Here's how the part is built. I have some questions about the finished solid (model axes, mm). A direction names the side the tool comes from. Coordinates: 2 decimals unless noted, no trailing zeros. Order: outer loops, then holes, each group sorted by start corner. A loop starts at its lowest first (then second) coordinate and runs counter-clockwise, first axis right, second up. Notation, with made-up numbers: (-28.75, 79.25) - (9.25, 79.25) arc R21 ccw to (9.25, 84.25) - close; hole circle Ø4 at (63, 49). An arc over 180 degrees is marked (long way). Answer as CSV lines item,"result". Start each with the question number.
Item 1: On a 3-axis mill with a long thin cutter (end or side, diameter ignored), from which of +Z, -Z, +X, -X, +Y, -Y can I reach the whole of each face in a straight line? I mean faces 1 (the face through (126, 2.478, 125)), 2 (the face through (0, -25, -20.408)), 3 (the face through (0, -12.729, 0)). Say none if no direction works.
Item 2: I need wall thicknesses on line 1 (X direction, y = 2, z = 37); line 2 (Y direction, x = 130, z = 122); line 3 (Y direction, x = 79, z = 74). Which ranges of each line are inside material? Lowest first, please.
Item 3: Imagine slicing it at B-B on z = 67. List the corners of the cut face in (x, y) for me.
Item 4: We'd pull the mould along X, two halves only. Please class faces 4 (the face through (22.5, -13, 2)), 5 (the face through (138.36, 4.94, -139.18)), 6 (the face through (0, -27.522, 0)), 7 (the face through (87.27, 1.21, -83.48)): pulls with the +X half, pulls with the -X half, needs draft (parallel to the pull), parting line crosses it, or undercut.
Item 5: I'm going to push flat-ended pins straight in: pin 1 (22 mm diameter, centred on y = -7, z = -6, fed in from -X); pin 2 (12 mm diameter, centred on y = -9.5, z = 32.5, fed in from -X); pin 3 (5 mm diameter, centred on y = -22.5, z = 5.5, fed in from +X); pin 4 (6 mm diameter, centred on x = 0, y = -21.5, fed in from -Z). Where does each tip first touch, or does it pass through?
Item 6: Imagine slicing it at A-A on z = 6. Count the separate pieces of the cut face and the enclosed holes in it, and give its area (3 significant figures).
from build123d import *

# Parameters (mm, degrees)
EXTRUDE_1_DEPTH     = 5
SKETCH_2_W          = 90
SKETCH_2_H          = 90
EXTRUDE_2_DEPTH     = 25
SKETCH_3_W          = 82.667839838
SKETCH_3_H          = 15.058257345
CUT_EXTRUDE_1_DEPTH = 90
SKETCH_4_W          = 82.085695662
SKETCH_4_H          = 16.995101666
CUT_EXTRUDE_2_DEPTH = 90
SKETCH_5_W          = 97.364780094
SKETCH_5_H          = 98.94366842
EXTRUDE_3_DEPTH     = 20
FILLET_1_R          = 10
SKETCH_6_W          = 90
SKETCH_6_H          = 90
EXTRUDE_4_DEPTH     = 30
CUT_EXTRUDE_3_DEPTH = 90
SKETCH_8_W          = 62.667839838
SKETCH_8_H          = 13.124346315
CUT_EXTRUDE_4_DEPTH = 10
CUT_EXTRUDE_5_DEPTH = 90
SKETCH_10_W         = 62.085695662
SKETCH_10_H         = 21.626220655
CUT_EXTRUDE_6_DEPTH = 10
SKETCH_11_W         = 62.667839838
SKETCH_11_H         = 13.124346315
CUT_EXTRUDE_7_DEPTH = 10
SKETCH_12_W         = 62.085695662
SKETCH_12_H         = 21.626220655
CUT_EXTRUDE_8_DEPTH = 10
EXTRUDE_5_DEPTH     = 20
SKETCH_14_R         = 25
EXTRUDE_6_DEPTH     = 20
FILLET_2_R          = 10
SCALE_1_SCALE       = 0.5


with BuildPart() as part:
    # 草图1 → 凸台-拉伸1 (new body)
    with BuildSketch(Plane(origin=(0, 0, 0), x_dir=(1, 0, 0), z_dir=(0, 1, 0))):
        Polygon((0, 70.903454713), (0, 0), (70.90345471, 0), (70.90345471, 50.896669322), (70.90345471, 63.546624398), (70.90345471, 70.903454713), (63.546624395, 70.903454713), (50.896669319, 70.903454713), align=None)
        Polygon((72.962659229, 92.969444623), (50.896669319, 70.903454713), (63.546624395, 70.903454713), (79.287636767, 86.644467085), align=None)
        Polygon((70.90345471, 70.903454713), (70.90345471, 63.546624398), (86.644467082, 79.28763677), (79.287636767, 86.644467085), (63.546624395, 70.903454713), align=None)
        Polygon((70.90345471, 63.546624398), (70.90345471, 50.896669322), (92.96944462, 72.962659232), (86.644467082, 79.28763677), align=None)
        with BuildLine():
            ThreePointArc((242.661241038, 250.018071355), (240.67172678, 254.833829646), (239.993214606, 260))
            Line((239.993214606, 260), (72.962659229, 92.969444623))
            Line((72.962659229, 92.969444623), (79.287636767, 86.644467085))
            Line((79.287636767, 86.644467085), (242.661241038, 250.018071355))
        make_face()
        with BuildLine():
            Line((92.96944462, 72.962659232), (260, 239.993214612))
            ThreePointArc((260, 239.993214606), (254.833829644, 240.67172678), (250.018071352, 242.66124104))
            Line((250.018071352, 242.66124104), (86.644467082, 79.28763677))
            Line((86.644467082, 79.28763677), (92.96944462, 72.962659232))
        make_face()
        with BuildLine():
            Line((260, 252.643169688), (260, 239.993214612))
            ThreePointArc((260, 239.993214606), (274.146933622, 245.853066378), (280.006785394, 260))
            ThreePointArc((280.006785394, 260), (260, 280.006785394), (239.993214606, 260))
            Line((239.993214606, 260), (252.643169682, 260))
            Line((252.643169682, 260), (260, 260))
            Line((260, 260), (260, 252.643169688))
        make_face()
        with BuildLine():
            Line((252.643169682, 260), (239.993214606, 260))
            ThreePointArc((239.993214606, 260), (240.67172678, 254.833829646), (242.661241038, 250.018071355))
            Line((242.661241038, 250.018071355), (252.643169682, 260))
        make_face()
        with BuildLine():
            ThreePointArc((250.018071352, 242.66124104), (254.833829644, 240.67172678), (260, 239.993214606))
            Line((260, 239.993214612), (260, 252.643169688))
            Line((260, 252.643169688), (250.018071352, 242.66124104))
        make_face()
    extrude_1 = extrude(amount=EXTRUDE_1_DEPTH)

    # 镜向1: 凸台-拉伸1 across plane
    add(extrude_1.mirror(Plane(origin=(0, 5, 0), x_dir=(0, 0, 1), z_dir=(1, 0, 0))))

    # 镜向3: part across plane


with BuildPart() as part_1:
    add(part.part)
    add(part.part.mirror(Plane(origin=(0, 5, 0), x_dir=(1, 0, 0), z_dir=(0, 0, -1))))

    # 草图2 → 凸台-拉伸2 (add)
    with BuildSketch(Plane.XZ):
        Rectangle(SKETCH_2_W, SKETCH_2_H)
    extrude(amount=EXTRUDE_2_DEPTH)

    # 草图3 → 切除-拉伸1 (cut)
    with BuildSketch(Plane.XY.offset(45)):
        with Locations((0, -12.246888496)):
            Rectangle(SKETCH_3_W, SKETCH_3_H)
    extrude(amount=-CUT_EXTRUDE_1_DEPTH, mode=Mode.SUBTRACT)

    # 草图4 → 切除-拉伸2 (cut)
    with BuildSketch(Plane(origin=(45, 0, 0), x_dir=(0, 0, -1), z_dir=(1, 0, 0))):
        with Locations((0, -12.272398252)):
            Rectangle(SKETCH_4_W, SKETCH_4_H)
    extrude(amount=-CUT_EXTRUDE_2_DEPTH, mode=Mode.SUBTRACT)

    # 草图5 → 凸台-拉伸3 (add)
    with BuildSketch(Plane(origin=(0, 5, 0), x_dir=(1, 0, 0), z_dir=(0, 1, 0))):
        Rectangle(SKETCH_5_W, SKETCH_5_H)
    extrude(amount=EXTRUDE_3_DEPTH)

    # 圆角1
    fillet_1_edges = [part_1.edges().sort_by_distance(p)[0] for p in [
        (48.682390047, 15, 49.47183421),
        (48.682390047, 15, -49.47183421),
        (-48.682390047, 15, -49.47183421),
        (-48.682390047, 15, 49.47183421),
        (48.682390047, 25, 0),
        (0, 25, -49.47183421),
        (-48.682390047, 25, 0),
        (0, 25, 49.47183421),
    ]]
    fillet(fillet_1_edges, radius=FILLET_1_R)

    # 草图6 → 凸台-拉伸4 (add)
    with BuildSketch(Plane.XZ.offset(25)):
        Rectangle(SKETCH_6_W, SKETCH_6_H)
    extrude(amount=EXTRUDE_4_DEPTH)

    # 草图7 → 切除-拉伸3 (cut)
    with BuildSketch(Plane.XY.offset(45)):
        Polygon((-41.333919919, -25.414932676), (41.333919919, -25.414932676), (41.333919919, -49.347564191), (31.333919919, -49.347564191), (31.333919919, -36.223217876), (-31.333919919, -36.223217876), (-31.333919919, -49.347564191), (-41.333919919, -49.347564191), align=None)
    extrude(amount=-CUT_EXTRUDE_3_DEPTH, mode=Mode.SUBTRACT)

    # 草图8 → 切除-拉伸4 (cut)
    with BuildSketch(Plane.XY.offset(45)):
        with Locations((0, -42.785391034)):
            Rectangle(SKETCH_8_W, SKETCH_8_H)
    extrude(amount=-CUT_EXTRUDE_4_DEPTH, mode=Mode.SUBTRACT)

    # 草图9 → 切除-拉伸5 (cut)
    with BuildSketch(Plane(origin=(45, 0, 0), x_dir=(0, 0, -1), z_dir=(1, 0, 0))):
        Polygon((-41.042847831, -26.273596919), (-41.042847831, -50.943507888), (-31.042847831, -50.943507888), (-31.042847831, -29.317287233), (31.042847831, -29.317287233), (31.042847831, -50.943507888), (41.042847831, -50.943507888), (41.042847831, -26.273596919), align=None)
    extrude(amount=-CUT_EXTRUDE_5_DEPTH, mode=Mode.SUBTRACT)

    # 草图10 → 切除-拉伸6 (cut)
    with BuildSketch(Plane(origin=(45, 0, 0), x_dir=(0, 0, -1), z_dir=(1, 0, 0))):
        with Locations((0, -40.130397561)):
            Rectangle(SKETCH_10_W, SKETCH_10_H)
    extrude(amount=-CUT_EXTRUDE_6_DEPTH, mode=Mode.SUBTRACT)

    # 草图11 → 切除-拉伸7 (cut)
    with BuildSketch(Plane(origin=(0, 0, -45), x_dir=(-1, 0, 0), z_dir=(0, 0, -1))):
        with Locations((0, -42.785391034)):
            Rectangle(SKETCH_11_W, SKETCH_11_H)
    extrude(amount=-CUT_EXTRUDE_7_DEPTH, mode=Mode.SUBTRACT)

    # 草图12 → 切除-拉伸8 (cut)
    with BuildSketch(Plane.ZY.offset(45)):
        with Locations((0, -40.130397561)):
            Rectangle(SKETCH_12_W, SKETCH_12_H)
    extrude(amount=-CUT_EXTRUDE_8_DEPTH, mode=Mode.SUBTRACT)

    # 草图13 → 凸台-拉伸5 (add)
    with BuildSketch(Plane.XY.offset(70.903454713)):
        Polygon((0, 0), (-10, 0), (-10, 5), (10, 5), (10, 0), align=None)
    extrude(amount=EXTRUDE_5_DEPTH)

    # 草图14 → 凸台-拉伸6 (add)
    with BuildSketch(Plane(origin=(0, 5, 0), x_dir=(1, 0, 0), z_dir=(0, 1, 0))):
        with Locations(Location((-260, 260, 0), (0, 0, 349.463237906))):
            Circle(SKETCH_14_R)
        with Locations(Location((260, 260, 0), (0, 0, 190.536762094))):
            Circle(SKETCH_14_R)
        with Locations(Location((-260, -260, 0), (0, 0, 79.463237895))):
            Circle(SKETCH_14_R)
        with Locations(Location((260, -260, 0), (0, 0, 100.536762105))):
            Circle(SKETCH_14_R)
    extrude(amount=EXTRUDE_6_DEPTH)

    # 圆角2
    fillet_2_edges = [part_1.edges().sort_by_distance(p)[0] for p in [
        (-284.578444482, 25, -264.571659088),
        (284.578444482, 25, -264.571659088),
        (-264.571659093, 25, 284.578444482),
        (264.571659093, 25, 284.578444482),
    ]]
    fillet(fillet_2_edges, radius=FILLET_2_R)


with BuildPart() as part_2:
    # 缩放比例1: scaled about (0, -0.043580376, 0.226767714)
    add(part_1.part.scale(SCALE_1_SCALE).moved(Location((0, -0.021790188, 0.113383857))))


solid = part_2.part
Responses:
1,face 1,"-Y"
1,face 2,"+X, -X"
1,face 3,"+Z, -Z"
2,line 1,"x = -46.89 to -26.88, -5 to 5, 26.88 to 46.89"
2,line 2,"y = -0.02 to 12.44"
2,line 3,"y = -0.02 to 2.48"
3,outline,"(-76.89, -0.02) - (-70.57, -0.02) - (-70.57, 2.48) - (-76.89, 2.48) - close; (-63.21, -0.02) - (-56.88, -0.02) - (-56.88, 2.48) - (-63.21, 2.48) - close; (56.88, -0.02) - (63.21, -0.02) - (63.21, 2.48) - (56.88, 2.48) - close; (70.57, -0.02) - (76.89, -0.02) - (76.89, 2.48) - (70.57, 2.48) - close"
4,face 4,"pulls with the +X half"
4,face 5,"undercut"
4,face 6,"needs draft"
4,face 7,"undercut"
5,pin 1,"stops at x = -35.45"
5,pin 2,"passes through"
5,pin 3,"stops at x = 17.5"
5,pin 4,"stops at z = -15.41"
6,separate pieces,"3"
6,enclosed holes,"0"
6,area,"1,170 mm^2"
